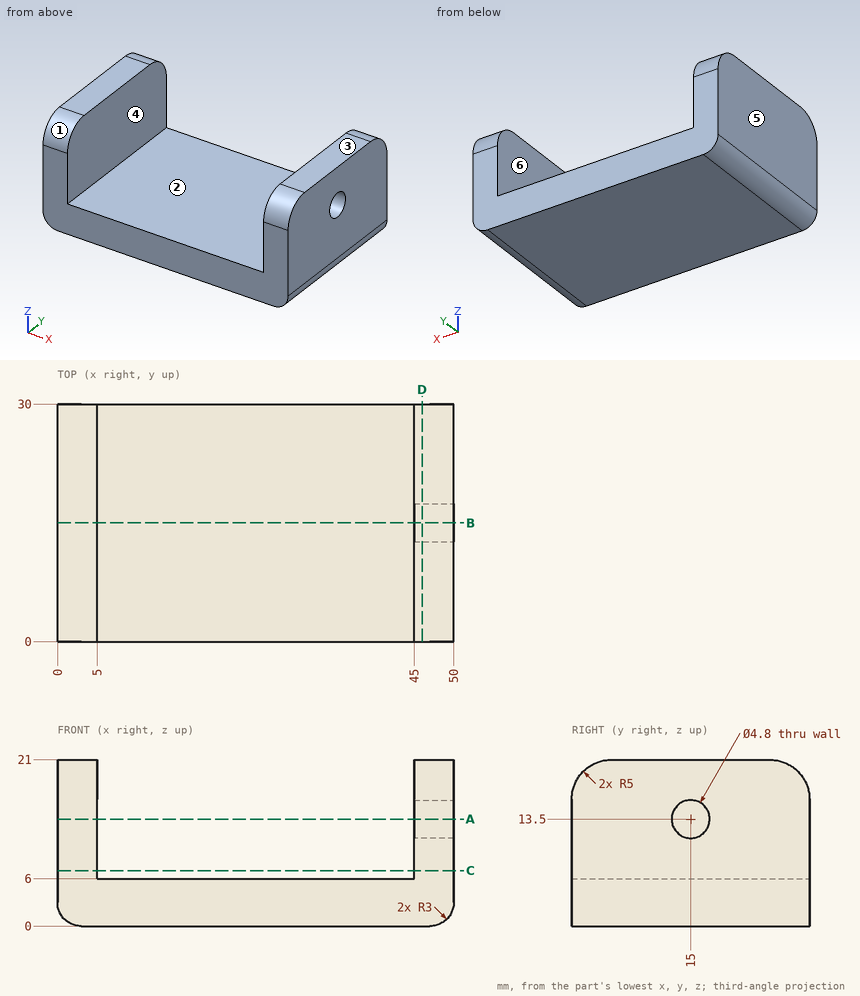
Can you work these out from the drawing? Everything is in mm from the part's minimum corner. A direction names the side the tool comes from. Give positions to 0.01 mm unless a question says otherwise; leave off trailing zeros. Order: outer loops, then holes, each group sorted by start corner. A loop starts at its lowest first (then second) coordinate and runs counter-clockwise, first axis right, second up. Notation, with made-up numbers: M -14,30.25 L -3,30.25 A13 cw -3,38.25 Z; hole C 9.5,-37 d5. An arc over 180 degrees is marked long. Use a Markdown table: item, result. Add a question column.
1. On a 3-axis mill with a long thin cutter (end or side, diameter ignored), from which of +Z, -Z, +X, -X, +Y, -Y can I reach the whole of each face in a straight line? I mean the marked faces 1 and 2. Say none if no direction works.
2. If we mould it in two halves opening along X, with no side actions, what happens to the marked faces 3, 4, 5 and 6? For each: +X half, -X half, draft (parallel to the pull), parting line (faces both ways), or undercut.
3. Suppose I cut it at B-B (y = 15). List the corners of the cut face in (x, z) for me, and give its area (3 significant figures).
4. I need wall thicknesses on probe 1 along X at (y, z) = (9.25, 15.25); probe 2 along Y at (x, z) = (47.3, 13.5); probe 3 along X at (y, z) = (13.5, 14.5). Which ranges of each line are inside material? Lowest first, please. Write a range as from..to.
5. Suppose I cut it at D-D (x = 46). List the corners of the cut face in (y, z) for me, and give its area (3 significant figures).
6. Suppose I cut it at A-A (z = 13.5). List the corners of the cut face in (x, y) for me, and give its area (3 significant figures).
7. For pin 1 Ø4 at (x, y) = (40, 6) entering from +Z; pin 2 Ø4 at (x, z) = (18, 9.5) entering from -Y, each with a flat end and sliding along its axis, tell me the tip position at first contact or that it passes through.
8. Suppose I cut it at C-C (z = 7). List the corners of the cut face in (x, y) for me.
Results list:
| question | item | result |
|---|---|---|
| 1 | face 1 | +Z, +X, -X, -Y |
| 1 | face 2 | +Z, +Y, -Y |
| 2 | face 3 | draft |
| 2 | face 4 | undercut |
| 2 | face 5 | -X half |
| 2 | face 6 | undercut |
| 3 | outline | M 0,3 A3 ccw 3,0 L 47,0 A3 ccw 50,3 L 50,11.1 L 45,11.1 L 45,6 L 5,6 L 5,21 L 0,21 Z; M 45,15.9 L 50,15.9 L 50,21 L 45,21 Z |
| 3 | area | 422 mm² |
| 4 | probe 1 | x = 0..5, 45..50 |
| 4 | probe 2 | y = 0..12.6, 17.4..30 |
| 4 | probe 3 | x = 0..5 |
| 5 | outline | M 0,0 L 30,0 L 30,16 A5 ccw 25,21 L 5,21 A5 ccw 0,16 Z; hole C 15,13.5 d4.8 |
| 5 | area | 601 mm² |
| 6 | outline | M 0,0 L 5,0 L 5,30 L 0,30 Z; M 45,0 L 50,0 L 50,12.6 L 45,12.6 Z; M 45,17.4 L 50,17.4 L 50,30 L 45,30 Z |
| 6 | area | 276 mm² |
| 7 | pin 1 | stops at z = 6 |
| 7 | pin 2 | passes through |
| 8 | outline | M 0,0 L 5,0 L 5,30 L 0,30 Z; M 45,0 L 50,0 L 50,30 L 45,30 Z |
